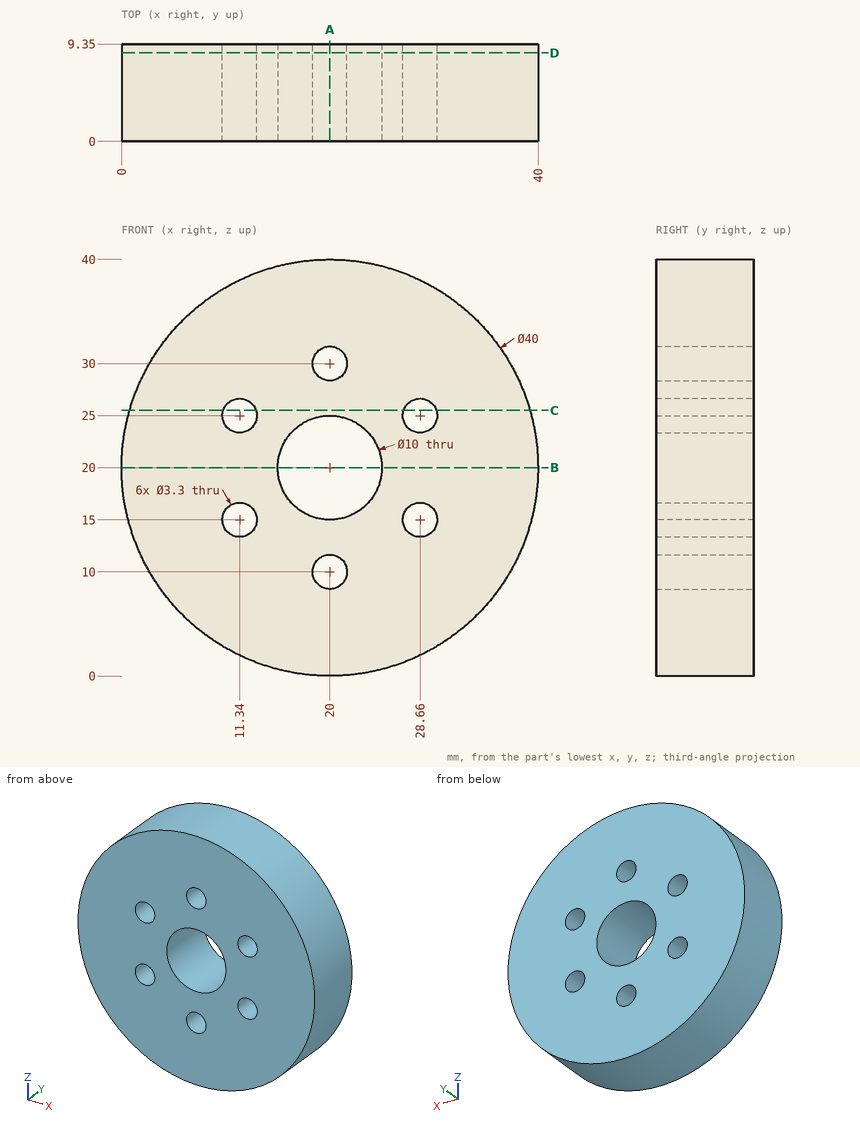
Drawing for the job (mm, zero at the part's lowest x, y, z). Coordinates: 2 decimals unless noted, no trailing zeros. Write each loop counter-clockwise with the first axis right and the second up, starting at its lowest first coordinate (ties: lowest second). Pieces come first, ordered by that corner, then holes. Notation, with made-up numbers: (23.5, 70) -> (67.5, 70) arc R22 ccw to (67.5, 83) -> close; hole circle Ø7 at (69, 45.5). An arc over 180 degrees is marked (long way). One line per item, written item: value. Start each with the question number.
1) Slice it at B-B on z = 20. Write the cut outline in (x, y).
2) Probe probe 1 along Z at (x, y) = (28, 4); probe 2 along Z at (x, y) = (11, 7.25) (1 decimal); probe 3 along X at (y, z) = (4.5, 10). List the from-to ranges inside material, lowest first.
3) Slice it at D-D on y = 8.5. Write the cut outline in (x, z), then the cut area to 3 significant figures.
4) Slice it at A-A on x = 20. Write the cut outline in (y, z), then the cut area to 3 significant figures.
5) Slice it at C-C on z = 25.5. Write the cut outline in (x, y), then the cut area to 3 significant figures.
6) Flat gauge pins, fed straight in: pin 1 Ø4 at (x, z) = (28.66, 15) entering from -Y; pin 2 Ø5 at (x, y) = (24, 6.5) entering from +Z; pin 3 Ø2 at (x, y) = (27.5, 7.5) entering from +Z; pin 4 Ø1 at (x, y) = (36, 5.5) entering from +Z. Where does each tip first touch, or does it go through?
Answers follow:
1. outline: (0, 0) -> (15, 0) -> (15, 9.35) -> (0, 9.35) -> close; (25, 0) -> (40, 0) -> (40, 9.35) -> (25, 9.35) -> close
2. probe 1: 1.67 to 13.49, 16.51 to 23.49, 26.51 to 38.33
2. probe 2: 2.1 to 13.4, 16.6 to 23.4, 26.6 to 37.9
2. probe 3: 2.68 to 18.35, 21.65 to 37.32
3. outline: circle Ø40 at (20, 20); hole circle Ø3.3 at (11.34, 15); hole circle Ø3.3 at (11.34, 25); hole circle Ø10 at (20, 20); hole circle Ø3.3 at (20, 10); hole circle Ø3.3 at (20, 30); hole circle Ø3.3 at (28.66, 15); hole circle Ø3.3 at (28.66, 25)
3. area: 1,130 mm2
4. outline: (0, 0) -> (9.35, 0) -> (9.35, 8.35) -> (0, 8.35) -> close; (0, 11.65) -> (9.35, 11.65) -> (9.35, 15) -> (0, 15) -> close; (0, 25) -> (9.35, 25) -> (9.35, 28.35) -> (0, 28.35) -> close; (0, 31.65) -> (9.35, 31.65) -> (9.35, 40) -> (0, 40) -> close
4. area: 219 mm2
5. outline: (0.77, 0) -> (9.77, 0) -> (9.77, 9.35) -> (0.77, 9.35) -> close; (12.91, 0) -> (27.09, 0) -> (27.09, 9.35) -> (12.91, 9.35) -> close; (30.23, 0) -> (39.23, 0) -> (39.23, 9.35) -> (30.23, 9.35) -> close
5. area: 301 mm2
6. pin 1: y = 0
6. pin 2: z = 39.94
6. pin 3: z = 38.91
6. pin 4: z = 32.64
